Answer from the drawing. Dimensions are ordinates in mm from the lowest x, y and z of the part. A direction names the side the tool comes from. Give positions to 0.01 mm unless a question says otherwise; leave off trailing zeros. Loops run counter-clockwise (first coordinate to the right, second up) from the corner with the lowest first, then second, coordinate; pieces in that order, holes last. Notation, with made-up numbers: (29.25, 38.5) -> (77.25, 38.5) arc R27 cw to (77.25, 58.5) -> close; hole circle Ø4 at (43.5, 25). An arc over 180 degrees is marked (long way). Return JSON: item names as keys, results as strings. Group by question number.
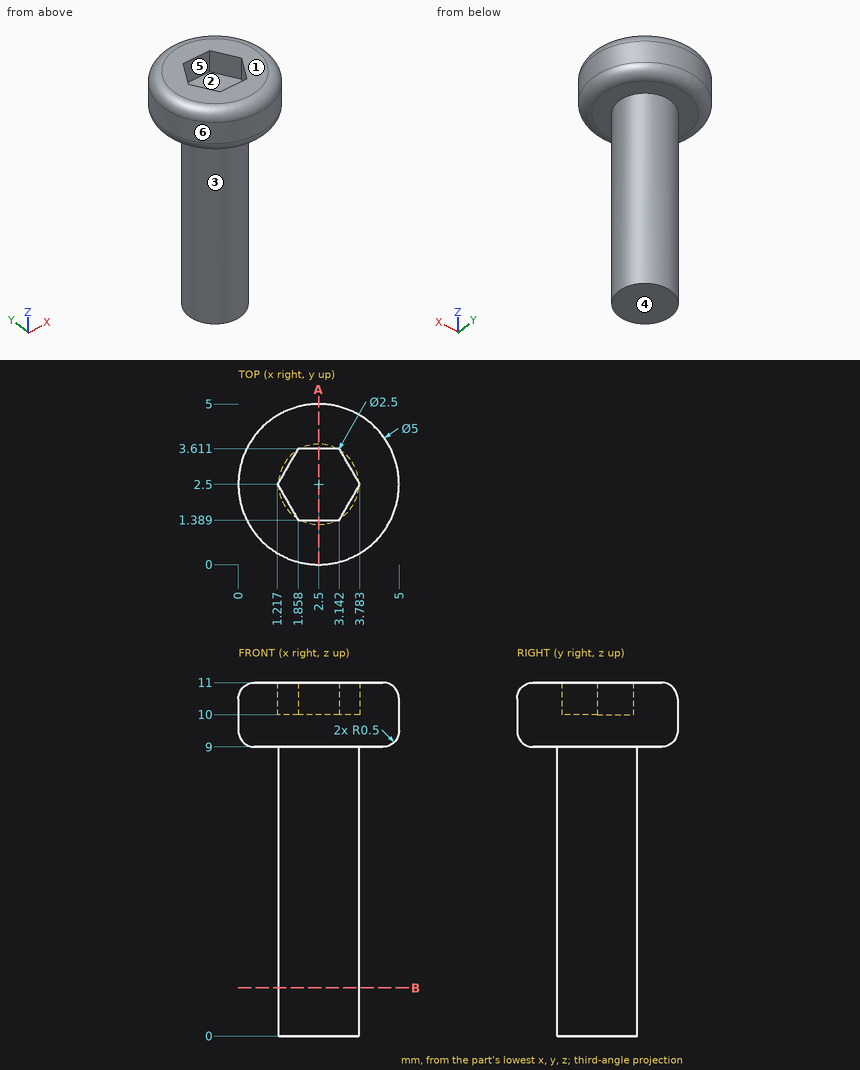
1. Straight lines are drawn through the part: line 1 (Z direction, x = 3.45, y = 4.3); line 2 (Z direction, x = 3.25, y = 2.95); line 3 (X direction, y = 2.45, z = 4). For each, find the intervals that lie inside material, in ascending order. Write a range as from..to.
2. Section B-B on z = 1.5 is taken. Determine the outline of the cut face in (x, y).
3. Flat-ended cylindrical pins translate along their axes: pin 1 Ø1.2 at (x, y) = (1.5, 2.5) entering from -Z; pin 2 Ø0.8 at (x, z) = (3, 10.5) entering from +Y; pin 3 Ø1.5 at (y, z) = (4, 9.5) entering from -X (1 decimal); pin 4 Ø1 at (x, z) = (3, 5.5) entering from -Y. Find the tip coordinate at first contact, or state that the pin passes through.
4. Which of the six approach directions +Z, -Z, +X, -X, +Y, -Y give full straight-line access (tool end or side, diameter ignored) to the marked faces 1, 2 and 3?
5. Determine the mould class of the marked faces 4, 5 and 6 for opening direction X: pulls with the +X half, pulls with the -X half, needs draft (parallel to the pull), parting line crosses it, or undercut.
6. Section A-A on x = 2.5 is taken. Determine the outline of the cut face in (y, z).
Completed:
{
 "1": {"line 1": "z = 9..11", "line 2": "z = 0..10", "line 3": "x = 1.25..3.75"},
 "2": {"outline": "circle Ø2.5 at (2.5, 2.5)"},
 "3": {"pin 1": "stops at z = 0", "pin 2": "stops at y = 5", "pin 3": "stops at x = 0.1", "pin 4": "stops at y = 1.25"},
 "4": {"face 1": "+Z, +X, -X, +Y, -Y", "face 2": "+Z", "face 3": "-Z"},
 "5": {"face 4": "needs draft", "face 5": "undercut", "face 6": "parting line crosses it"},
 "6": {"outline": "(0, 9.5) arc R0.5 ccw to (0.5, 9) -> (1.25, 9) -> (1.25, 0) -> (3.75, 0) -> (3.75, 9) -> (4.5, 9) arc R0.5 ccw to (5, 9.5) -> (5, 10.5) arc R0.5 ccw to (4.5, 11) -> (3.61, 11) -> (3.61, 10) -> (1.39, 10) -> (1.39, 11) -> (0.5, 11) arc R0.5 ccw to (0, 10.5) -> close"}
}
